```python
from build123d import *

# Parameters (mm, degrees)
F0_R      = 16.999966
F1_DEPTH  = 3.999992
F2_R      = 14
F2_R_2    = 12
F3_DEPTH  = 0.25
F4_DEPTH  = 1
F5_R      = 5.5
F6_DEPTH  = 1
F7_R      = 2.5
F8_DEPTH  = 2
F9_R      = 0.5
F11_DEPTH = 0.5
F10_R     = 2
F12_DEPTH = 25
F13_R     = 14
F13_R_2   = 12
F14_DEPTH = 0.25
F15_DEPTH = 1
F16_R     = 3
F16_R_2   = 1.5
F17_DEPTH = 11


with BuildPart() as f1:
    # F0 (on Front) → F1 (new body)
    with BuildSketch(Plane.XZ):
        with Locations((-39.9907566607, 30.1120206714)):
            Circle(F0_R)
    extrude(amount=F1_DEPTH)

    # F2 (on face) → F3 (cut)
    with BuildSketch(Plane.XZ.offset(3.999992)):
        with Locations((-39.9907566607, 30.1120206714)):
            Circle(F2_R)
        with Locations((-39.9907566607, 30.1120206714)):
            Circle(F2_R_2, mode=Mode.SUBTRACT)
    extrude(amount=-F3_DEPTH, mode=Mode.SUBTRACT)

    # F4 (cut): a face of the model
    f4_faces = [f1.faces().sort_by_distance(p)[0] for p in [
        (-39.9907566607, -3.999992, 30.1120206714),
    ]]
    extrude(f4_faces, amount=-F4_DEPTH, mode=Mode.SUBTRACT)

    # F5 (on face) → F6 (join)
    with BuildSketch(Plane.XZ.offset(2.999992)):
        with Locations((-39.9907566607, 30.1120206714)):
            Circle(F5_R)
    extrude(amount=F6_DEPTH)

    # F7 (on face) → F8 (join)
    with BuildSketch(Plane.XZ.offset(3.999992)):
        with Locations((-39.9907566607, 30.1120206714)):
            Circle(F7_R)
    extrude(amount=F8_DEPTH)

    # F9 (on face) → F11 (join)
    with BuildSketch(Plane.XZ.offset(3.999992)):
        with Locations((-37.9335082777, 32.9435801517)):
            Circle(F9_R)
        with Locations((-39.9907566607, 33.6120206714)):
            Circle(F9_R)
        with Locations((-42.0480050437, 32.9435801517)):
            Circle(F9_R)
        with Locations((-43.3194544677, 31.1935801517)):
            Circle(F9_R)
        with Locations((-43.3194544677, 29.0304611911)):
            Circle(F9_R)
        with Locations((-42.0480050437, 27.2804611911)):
            Circle(F9_R)
        with Locations((-39.9907566607, 26.6120206714)):
            Circle(F9_R)
        with Locations((-37.9335082777, 27.2804611911)):
            Circle(F9_R)
        with Locations((-36.6620588537, 29.0304611911)):
            Circle(F9_R)
        with Locations((-36.6620588537, 31.1935801517)):
            Circle(F9_R)
    extrude(amount=F11_DEPTH)

    # F10 (on face) → F12 (cut)
    with BuildSketch(Plane.XZ.offset(2.999992)):
        with Locations((-33.5699219599, 23.8027328735)):
            Circle(F10_R)
        with Locations((-39.9118810892, 21.1104647272)):
            Circle(F10_R)
        with Locations((-46.3000444586, 23.6911859705)):
            Circle(F10_R)
        with Locations((-48.9923126049, 30.0331450999)):
            Circle(F10_R)
        with Locations((-46.4115913615, 36.4213084693)):
            Circle(F10_R)
        with Locations((-40.0696322322, 39.1135766156)):
            Circle(F10_R)
        with Locations((-33.6814688628, 36.5328553722)):
            Circle(F10_R)
        with Locations((-30.9892007165, 30.1908962429)):
            Circle(F10_R)
    extrude(amount=-F12_DEPTH, mode=Mode.SUBTRACT)

    # F13 (on face) → F14 (cut)
    with BuildSketch(Plane(origin=(0, 0, 0), x_dir=(-1, 0, 0), z_dir=(0, 1, 0))):
        with Locations((39.9907566607, 30.1120206714)):
            Circle(F13_R)
        with Locations((39.9907566607, 30.1120206714)):
            Circle(F13_R_2, mode=Mode.SUBTRACT)
    extrude(amount=-F14_DEPTH, mode=Mode.SUBTRACT)

    # F15 (cut): a face of the model
    f15_faces = [f1.faces().sort_by_distance(p)[0] for p in [
        (-39.9907566607, 0, 30.1120206714),
    ]]
    extrude(f15_faces, amount=-F15_DEPTH, mode=Mode.SUBTRACT)

    # F16 (on face) → F17 (join)
    with BuildSketch(Plane(origin=(0, -1, 0), x_dir=(-1, 0, 0), z_dir=(0, 1, 0))):
        with Locations((39.9907566607, 30.1120206714)):
            Circle(F16_R)
        with Locations((39.9907566607, 30.1120206714)):
            Circle(F16_R_2, mode=Mode.SUBTRACT)
    extrude(amount=F17_DEPTH)


solid = f1.part
```
Check sheet for the modelled part. Datum: model origin and axes. Units: mm. A direction names the side the tool comes from. Round coordinates to 2 decimals unless told otherwise and drop trailing zeros. Order: outer loops, then holes, each group sorted by start corner. A loop starts at its lowest first (then second) coordinate and runs counter-clockwise, first axis right, second up. Notation, with made-up numbers: (39, -30.75) - (69, -30.75) arc R9 ccw to (69, -24.75) - close; hole circle Ø4 at (35.5, 51). An arc over 180 degrees is marked (long way). Answer as CSV lines item,"result". Start each with the question number.
1) Depth check by flat-ended pin: pin 1 (0.5 mm diameter, centred on x = -36.5, z = 31.5, fed in from -Y); pin 2 (3 mm diameter, centred on x = -28, y = -3.5, fed in from +Z); pin 3 (2 mm diameter, centred on y = 8, z = 31.5, fed in from -X). Enter the tip coordinate at first touch or a pass-through.
2) Section check B-B (z = 35). Give the number of separate pieces and of enclosed holes in the cut face, then the cut area to 3 significant figures.
3) Scan lines: probe 1 along Z at (x, y) = (-35, -2.25); probe 2 along X at (y, z) = (6.25, 30); probe 3 along Y at (x, z) = (-52.5, 34.5). Record each from-to range of solid material in increasing order.
4) Section check D-D (z = 43). Record the cut outline in (x, y), then the cut area to 3 significant figures.
5) Section check A-A (x = -30). Record the cut outline in (y, z).
6) Section check C-C (x = -46). Record the cut outline in (y, z), then the cut area to 3 significant figures.
7) Draft check along Z on faces 1 (the face through (-56.974, -1.972, 30.859)), 2 (the face through (-42, -4.5, 27)), 3 (the face through (-37, -1, 28)). Enter one of: +Z half, -Z half, draft (parallel to the pull), parting line (faces both ways), or undercut.
8) Tool access check on faces 4 (the face through (-40, -4.5, 26.6)), 5 (the face through (-42.445, -4.246, 32.639)), 6 (the face through (-40, -1, 30)), 7 (the face through (-40, -4.5, 33.6)). Record the directions out of +Z, -Z, +X, -X, +Y, -Y that give a thin tool (end or side, any length) a straight path to the whole face; none if there is none.
Determined:
1,pin 1,"y = -4.5"
1,pin 2,"z = 43.49"
1,pin 3,"x = -42.97"
2,separate pieces,"3"
2,enclosed holes,"0"
2,area,"78.5 mm^2"
3,probe 1,"13.86 to 22.4, 25.2 to 35.03, 38.04 to 46.36"
3,probe 2,"-42.99 to -41.49, -38.49 to -36.99"
3,probe 3,"-3.75 to -0.25"
4,outline,"(-51.08, -4) - (-45.46, -4) - (-45.46, -3.75) - (-34.52, -3.75) - (-34.52, -4) - (-28.9, -4) - (-28.9, 0) - (-34.52, 0) - (-34.52, -0.25) - (-45.46, -0.25) - (-45.46, 0) - (-51.08, 0) - close"
4,area,"83.2 mm^2"
5,outline,"(-4, 16.36) - (0, 16.36) - (0, 20.3) - (-0.25, 20.3) - (-0.25, 23.46) - (-1, 23.46) - (-1, 28.45) - (-3, 28.45) - (-3, 23.46) - (-3.75, 23.46) - (-3.75, 20.3) - (-4, 20.3) - close; (-4, 39.92) - (-3.75, 39.92) - (-3.75, 36.76) - (-3, 36.76) - (-3, 31.93) - (-1, 31.93) - (-1, 36.76) - (-0.25, 36.76) - (-0.25, 39.92) - (0, 39.92) - (0, 43.87) - (-4, 43.87) - close"
6,outline,"(-4, 14.21) - (0, 14.21) - (0, 17.47) - (-0.25, 17.47) - (-0.25, 19.73) - (-1, 19.73) - (-1, 21.71) - (-3, 21.71) - (-3, 19.73) - (-3.75, 19.73) - (-3.75, 17.47) - (-4, 17.47) - close; (-4, 42.76) - (-3.75, 42.76) - (-3.75, 40.5) - (-3, 40.5) - (-3, 38.38) - (-1, 38.38) - (-1, 40.5) - (-0.25, 40.5) - (-0.25, 42.76) - (0, 42.76) - (0, 46.01) - (-4, 46.01) - close; (-3, 25.67) - (-1, 25.67) - (-1, 34.46) - (-3, 34.46) - close"
6,area,"67.7 mm^2"
7,face 1,"parting line"
7,face 2,"draft"
7,face 3,"undercut"
8,face 4,"-Z, +X, -X, -Y"
8,face 5,"-Y"
8,face 6,"+Y"
8,face 7,"+Z, +X, -X, -Y"
